Check sheet for the modelled part. Datum: model origin and axes. Units: mm. Give positions to 0.01 mm unless a question says otherwise; leave off trailing zeros. Write each loop counter-clockwise with the first axis right and the second up, starting at its lowest first coordinate (ties: lowest second). Pieces come first, ordered by that corner, then holes. Notation, with made-up numbers: M 70,55.25 L 113,55.25 A14 cw 113,65.25 Z; hole C 76.5,72 d1. An arc over 180 degrees is marked long. One line per item, written item: value. Start each with the question number.
from build123d import *

# Parameters (mm, degrees)
BOSS_EXTRUDE1_DEPTH   = 7.62
LPATTERN2_COUNT       = 2
LPATTERN2_PITCH       = 53.34
BODY_MOVE_COPY1_ANGLE = 180
LPATTERN3_COUNT       = 3
LPATTERN3_PITCH       = 146.05
BODY_MOVE_COPY2_ANGLE = 120
BODY_MOVE_COPY3_ANGLE = 120
BOSS_EXTRUDE2_START   = 57.15
SKETCH2_R             = 9.5
BOSS_EXTRUDE2_DEPTH   = 486.09


with BuildPart() as part:
    # Sketch1 → Boss-Extrude1 (new body)
    with BuildSketch(Plane(origin=(0, 0, 0), x_dir=(1, 0, 0), z_dir=(0, 1, 0))):
        with BuildLine():
            Line((-5.499261314, 15.875), (-10.998522628, 6.35))
            ThreePointArc((-10.998522628, 6.35), (0, -12.7), (10.998522628, 6.35))
            Line((10.998522628, 6.35), (5.499261314, 15.875))
            ThreePointArc((5.499261314, 15.875), (0, 19.05), (-5.499261314, 15.875))
        make_face()
    extrude(amount=BOSS_EXTRUDE1_DEPTH)


with BuildPart() as lpattern2_1:
    # LPattern2: pattern copy
    add(part.part.moved(Location(Vector(0, -1, 0) * (1 * LPATTERN2_PITCH))))


with BuildPart() as lpattern2_1_1:
    # Body-Move_Copy1: moved
    add(lpattern2_1.part.rotate(Axis((0, 0, 0), (0, 1, 0)), BODY_MOVE_COPY1_ANGLE))


with BuildPart() as lpattern3_1:
    # LPattern3: pattern copy
    add(part.part.moved(Location(Vector(0, -1, 0) * (1 * LPATTERN3_PITCH))))


with BuildPart() as lpattern3_2:
    # LPattern3: pattern copy
    add(part.part.moved(Location(Vector(0, -1, 0) * (2 * LPATTERN3_PITCH))))


with BuildPart() as lpattern3_3:
    # LPattern3: pattern copy
    add(lpattern2_1_1.part.moved(Location(Vector(0, -1, 0) * (1 * LPATTERN3_PITCH))))


with BuildPart() as lpattern3_4:
    # LPattern3: pattern copy
    add(lpattern2_1_1.part.moved(Location(Vector(0, -1, 0) * (2 * LPATTERN3_PITCH))))


with BuildPart() as lpattern3_1_1:
    # Body-Move_Copy2: moved
    add(lpattern3_1.part.rotate(Axis((0, 0, 0), (0, -1, 0)), BODY_MOVE_COPY2_ANGLE))


with BuildPart() as lpattern3_3_1:
    # Body-Move_Copy2: moved
    add(lpattern3_3.part.rotate(Axis((0, 0, 0), (0, -1, 0)), BODY_MOVE_COPY2_ANGLE))


with BuildPart() as lpattern3_2_1:
    # Body-Move_Copy3: moved
    add(lpattern3_2.part.rotate(Axis((0, 0, 0), (0, 1, 0)), BODY_MOVE_COPY3_ANGLE))


with BuildPart() as lpattern3_4_1:
    # Body-Move_Copy3: moved
    add(lpattern3_4.part.rotate(Axis((0, 0, 0), (0, 1, 0)), BODY_MOVE_COPY3_ANGLE))


with BuildPart() as part_1:
    add(part.part)

    add(lpattern2_1_1.part)  # Boss-Extrude2 merges LPattern2_1

    add(lpattern3_1_1.part)  # Boss-Extrude2 merges LPattern3_1

    add(lpattern3_2_1.part)  # Boss-Extrude2 merges LPattern3_2

    add(lpattern3_3_1.part)  # Boss-Extrude2 merges LPattern3_3

    add(lpattern3_4_1.part)  # Boss-Extrude2 merges LPattern3_4
    # Sketch2 → Boss-Extrude2 (add)
    with BuildSketch(Plane(origin=(0, 0, 0), x_dir=(1, 0, 0), z_dir=(0, 1, 0)).offset(BOSS_EXTRUDE2_START)):
        with Locations(Location((0, 0, 0), (0, 0, 270))):
            Circle(SKETCH2_R)
    extrude(amount=-BOSS_EXTRUDE2_DEPTH)


solid = part_1.part
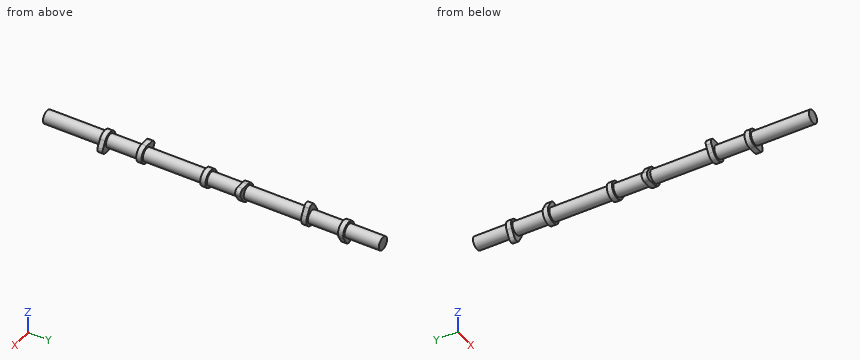
1) Gauge pin test, flat ends, axial feed: pin 1 (3 mm diameter, centred on x = 10.5, z = 6.5, fed in from +Y); pin 2 (5 mm diameter, centred on y = -98.5, z = 5, fed in from -X); pin 3 (1 mm diameter, centred on y = -84, z = -1, fed in from +X). Record the tip position at first contact, or that the pin passes through.
2) Cross-section at A-A (y = 12). Record the boundary of the cut face in (x, z), plus the area to 3 significant figures.
3) Material ranges on L1, parallel to Y at x = -9.5, z = 7.5; L2, parallel to X at y = -285.5, z = 6.5; L3, parallel to X at y = -193.5, z = 11, recorded low to high. Write a range as from..to.
Data:
1. pin 1: stops at y = 7.62
1. pin 2: stops at x = -9.17
1. pin 3: stops at x = 9.49
2. outline: C 0,0 d19
2. area: 284 mm2
3. L1: y = -345.44..-337.82, -292.1..-284.48, -199.39..-191.77, -146.05..-138.43, -53.34..-45.72, 0..7.62
3. L2: x = -17.35..10.91
3. L3: x = -6.35..6.35
